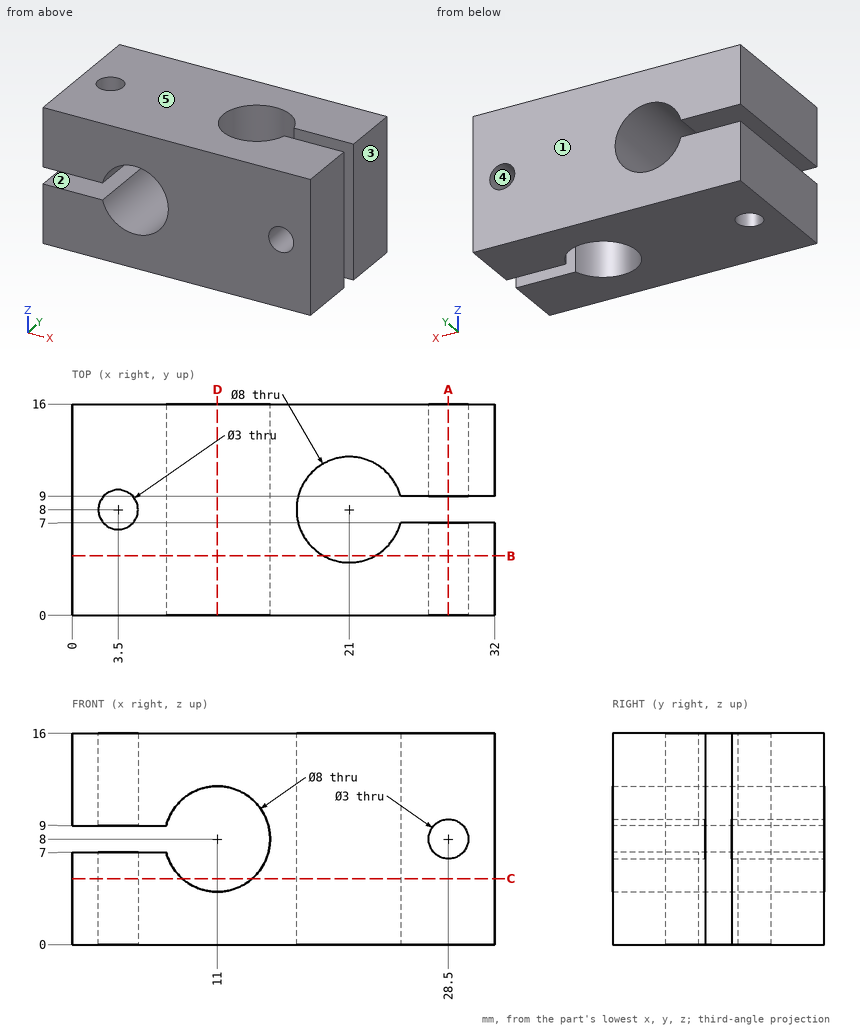
Can you work these out from the drawing? Everything is in mm from the part's minimum corner. A direction names the side the tool comes from. Give positions to 0.01 mm unless a question says otherwise; leave off trailing zeros. Loops run counter-clockwise (first coordinate to the right, second up) from the corner with the lowest first, then second, coordinate; pieces in that order, holes last. Notation, with made-up numbers: (53, 32) - (96, 32) arc R27 cw to (96, 55) - close; hole circle Ø6 at (56, 87). An arc over 180 degrees is marked (long way). Answer as a JSON object with one key per item and string values.
Q1. Imagine slicing it at C-C on z = 5. Write out the boundary of the cut face in (x, y), plus the area to 3 significant figures.
Geometry says:
{"outline": "(0, 0) - (8.35, 0) - (8.35, 16) - (0, 16) - close; (13.65, 0) - (32, 0) - (32, 7) - (24.87, 7) arc R4 cw (long way) to (24.87, 9) - (32, 9) - (32, 16) - (13.65, 16) - close; hole circle Ø3 at (3.5, 8)", "area": "356 mm²"}
Q2. Which directions (+Z, -Z, +X, -X, +Y, -Y) give clear straight access to the entire face, cutting with the end or side of a thin tool? Please do the marked faces 1 and 2.
Geometry says:
{"face 1": "+Z, -Z, +X, -X, +Y", "face 2": "-X, +Y, -Y"}
Q3. Imagine slicing it at B-B on y = 4.5. Write out the boundary of the cut face in (x, z).
Geometry says:
{"outline": "(0, 0) - (19.06, 0) - (19.06, 16) - (0, 16) - (0, 9) - (7.13, 9) arc R4 cw (long way) to (7.13, 7) - (0, 7) - close; (22.94, 0) - (32, 0) - (32, 16) - (22.94, 16) - close; hole circle Ø3 at (28.5, 8)"}
Q4. Imagine slicing it at A-A on x = 28.5. Write out the boundary of the cut face in (y, z).
Geometry says:
{"outline": "(0, 0) - (7, 0) - (7, 6.5) - (0, 6.5) - close; (0, 9.5) - (7, 9.5) - (7, 16) - (0, 16) - close; (9, 0) - (16, 0) - (16, 6.5) - (9, 6.5) - close; (9, 9.5) - (16, 9.5) - (16, 16) - (9, 16) - close"}
Q5. If we mould it in two halves opening along X, with no side actions, what happens to the marked faces 3, 4 and 5? For each: pulls with the +X half, pulls with the -X half, needs draft (parallel to the pull), parting line crosses it, or undercut.
Geometry says:
{"face 3": "pulls with the +X half", "face 4": "undercut", "face 5": "needs draft"}
Q6. If I drill on L1, parallel to Y at x = 3.5, z = 11; L2, parallel to Z at x = 3.5, y = 4.25; L3, parallel to Z at x = 11, y = 8.5, over which ranges is the centre line in solid material (lowest first)?
Geometry says:
{"L1": "0 to 6.5, 9.5 to 16", "L2": "0 to 7, 9 to 16", "L3": "0 to 4, 12 to 16"}
Q7. Will this pin go through, and if not, where does the flat tip stop? P1, Ø5.5, axis at x = 2.5, y = 7, coming from the +Z side.
Geometry says:
{"P1": "z = 16"}
Q8. Imagine slicing it at D-D on x = 11. Write out the boundary of the cut face in (y, z).
Geometry says:
{"outline": "(0, 0) - (16, 0) - (16, 4) - (0, 4) - close; (0, 12) - (16, 12) - (16, 16) - (0, 16) - close"}
